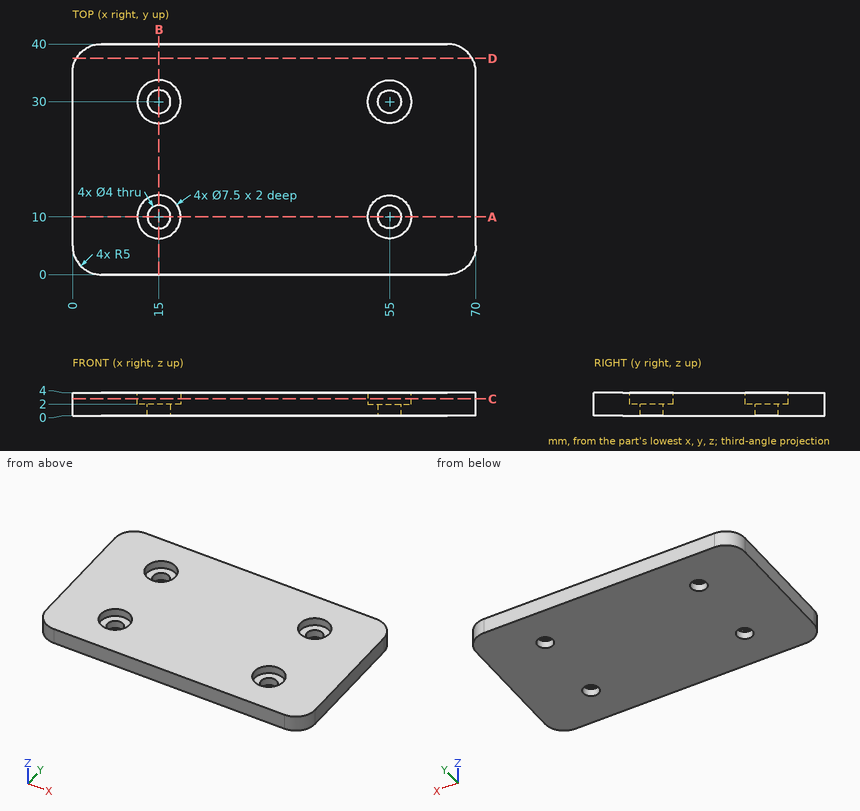
Could you check a few things on this drawing? It's one solid part, dimensions in mm from its lowest x, y, z. Coordinates: 2 decimals unless noted, no trailing zeros. Write each loop counter-clockwise with the first axis right and the second up, starting at its lowest first coordinate (ties: lowest second). Pieces come first, ordered by that corner, then holes. Notation, with made-up numbers: (31, 62) - (50, 62) arc R15 cw to (50, 79) - close; hole circle Ø11 at (80.5, -1.5). An arc over 180 degrees is marked (long way). Use one line per item in the form item = value.
1) I need wall thicknesses on line 1 (Y direction, x = 15, z = 0.95); line 2 (Y direction, x = 18, z = 2.7); line 3 (X direction, y = 12, z = 3.8). Which ranges of each line are inside material? Lowest first, please.
Solved:
line_1 = 0 to 8, 12 to 28, 32 to 40
line_2 = 0 to 7.75, 12.25 to 27.75, 32.25 to 40
line_3 = 0 to 11.83, 18.17 to 51.83, 58.17 to 70
2) I'm going to push a flat-ended pin straight in: P1, Ø4, axis at x = 15, y = 31, coming from the +Z side. Where does the tip first touch, or does it pass through?
Solved:
P1 = 2
3) Suppose I cut it at D-D, the plane y = 37.5. Write out the boundary of the cut face in (x, z), plus the area to 3 significant figures.
Solved:
outline = (0.67, 0) - (69.33, 0) - (69.33, 4) - (0.67, 4) - close
area = 275 mm2
4) Suppose I cut it at A-A, the plane y = 10. Write out the boundary of the cut face in (x, z).
Solved:
outline = (0, 0) - (13, 0) - (13, 2) - (11.25, 2) - (11.25, 4) - (0, 4) - close; (17, 0) - (53, 0) - (53, 2) - (51.25, 2) - (51.25, 4) - (18.75, 4) - (18.75, 2) - (17, 2) - close; (57, 0) - (70, 0) - (70, 4) - (58.75, 4) - (58.75, 2) - (57, 2) - close
5) Suppose I cut it at B-B, the plane x = 15. Write out the boundary of the cut face in (y, z), plus the area to 3 significant figures.
Solved:
outline = (0, 0) - (8, 0) - (8, 2) - (6.25, 2) - (6.25, 4) - (0, 4) - close; (12, 0) - (28, 0) - (28, 2) - (26.25, 2) - (26.25, 4) - (13.75, 4) - (13.75, 2) - (12, 2) - close; (32, 0) - (40, 0) - (40, 4) - (33.75, 4) - (33.75, 2) - (32, 2) - close
area = 114 mm2
6) Suppose I cut it at C-C, the plane z = 2.9. Write out the boundary of the cut face in (x, y), plus the area to 3 significant figures.
Solved:
outline = (0, 5) arc R5 ccw to (5, 0) - (65, 0) arc R5 ccw to (70, 5) - (70, 35) arc R5 ccw to (65, 40) - (5, 40) arc R5 ccw to (0, 35) - close; hole circle Ø7.5 at (15, 10); hole circle Ø7.5 at (15, 30); hole circle Ø7.5 at (55, 10); hole circle Ø7.5 at (55, 30)
area = 2,600 mm2
